Geometry check sheet. Reference: the model listing, model coordinates, mm. A direction names the side the tool comes from. Give positions to 0.01 mm unless a question says otherwise; leave off trailing zeros. Order: outer loops, then holes, each group sorted by start corner. A loop starts at its lowest first (then second) coordinate and runs counter-clockwise, first axis right, second up. Notation, with made-up numbers: M -34,-34.5 L -10,-34.5 A17 ccw -10,-5.5 Z; hole C -7.75,47 d2. An arc over 180 degrees is marked long. One line per question, with ' | ' between items. Start each with the question number.
Autodesk Inventor part; units mm, degrees
ref_plane "YZ Plane" through (0, 0, 0) normal (1, 0, 0) x (0, 1, 0)
ref_plane "XZ Plane" through (0, 0, 0) normal (0, 1, 0) x (-1, 0, 0)
ref_plane "XY Plane" through (0, 0, 0) normal (0, 0, 1) x (1, 0, 0)
sketch "Sketch1" plane through (0, 0, 0) normal (0, 0, 1) x (1, 0, 0)
  circle A0 centre (0, 0) radius 7.5
  arc A1 (6, -6.5) -> (6, 6.5) centre (6, 0) ccw
  line L0 (6, -6.5) -> (-6, -6.5)
  arc A2 (-6, 6.5) -> (-6, -6.5) centre (-6, 0) ccw
  line L1 (-6, 6.5) -> (6, 6.5)
  dimension "d0" = 15
  dimension "d6" = 6
  dimension "d8" = 6
  dimension "d22" = 6.5
  dimension "d23" = 6.5
  dimension "d24" = 12
extrude "Extrusion1" add sketch "Sketch1" along normal blind 3
sketch "草圖4" plane through (0, 0, 3) normal (0, 0, 1) x (1, 0, 0)
  arc A0 (3.7417, 6.5) -> (-3.7417, 6.5) centre (0, 0) ccw
  line L0 (1.3279, 2.3) -> (2.6558, 0)
  line L1 (2.6558, 0) -> (1.3279, -2.3)
  line L2 (1.3279, -2.3) -> (-1.3279, -2.3)
  line L3 (-1.3279, -2.3) -> (-2.6558, 0)
  line L4 (-2.6558, 0) -> (-1.3279, 2.3)
  line L5 (-1.3279, 2.3) -> (1.3279, 2.3)
  point P0 (-2.7439, 4.7667)
  point P1 (2.7439, 4.7667)
  point P2 (-6, -4.5)
  point P3 (6, -4.5)
  dimension "d17" = 4.6
extrude "擠出2" cut sketch "草圖4" against normal through all
fillet "圓角2" radius 4 4 edges at (3.7417, -6.5, 1.5) (-3.7417, -6.5, 1.5) (3.7417, 6.5, 1.5) (-3.7417, 6.5, 1.5)
sketch "草圖5" plane through (0, 0, 3) normal (0, 0, 1) x (1, 0, 0)
  arc A0 (6, -6.5) -> (6, 6.5) centre (6, 0) ccw
  arc A1 (-6, 6.5) -> (-6, -6.5) centre (-6, 0) ccw
hole "孔2" at (-6, 0, 3) at (6, 0, 3) direction (0, 0, -1) diameter 3 end through all
properties part number "plastic_part_99"
Item 1: Cross-section at D-D, the plane x = 10.5. Record the cut outline in (y, z), plus the area to 3 significant figures.
Item 2: Cross-section at A-A, the plane z = 1.55. Record the cut outline in (x, y), plus the area to 3 significant figures.
Item 3: Cross-section at C-C, the plane x = -1.75. Record the cut outline in (y, z).
Item 4: Material ranges on line 1 along Y through (x, z) = (-6, 2.1); line 2 along X through (y, z) = (0.5, 2.05); line 3 along Y through (x, z) = (1.5, 1.85), recorded low to high.
Item 5: Depth check by flat-ended pin: pin 1 (1.4 mm diameter, centred on x = 5, z = 1.5, fed in from +Y); pin 2 (1.4 mm diameter, centred on x = 5, z = 1, fed in from -Y). Enter the tip coordinate at first touch or a pass-through.
Item 6: Cross-section at B-B, the plane y = 1.25. Record the cut outline in (x, z), plus the area to 3 significant figures.
Item 7: Set-up check for faces 4 (the flat face through (5, 6.5, 1)), 5 (the flat face through (-2.001, 1.134, 1.521)), 6 (the flat face through (-5, -6.5, 1)): record each of +Z, -Z, +X, -X, +Y, -Y from which the full face is reachable in a straight line by a thin tool's end or side.
Item 8: Mould release check, pull along X, two halves, no side actions. Record for faces 1 (the cylindrical face through (3.8, 6.6, 1.5)), 2 (the flat face through (-3, 0, 0)), 3 (the cylindrical face through (7.464, 0.325, 1.479)): released by +X, released by -X, zero draft, split by the parting line, or undercut.
Outcome:
1) outline: M -4.69,0 L 4.69,0 L 4.69,3 L -4.69,3 Z | area: 28.1 mm²
2) outline: M -6,-6.5 L -4.69,-6.5 A4 cw -3.06,-6.85 A7.5 ccw 3.06,-6.85 A4 cw 4.69,-6.5 L 6,-6.5 A6.5 ccw 6,6.5 L 4.69,6.5 A4 cw 3.06,6.85 A7.5 ccw -3.06,6.85 A4 cw -4.69,6.5 L -6,6.5 A6.5 ccw Z; hole C -6,0 d3; hole M -2.66,0 L -1.33,-2.3 L 1.33,-2.3 L 2.66,0 L 1.33,2.3 L -1.33,2.3 Z; hole C 6,0 d3 | area: 267 mm²
3) outline: M -7.29,0 L -1.57,0 L -1.57,3 L -7.29,3 Z; M 1.57,0 L 7.29,0 L 7.29,3 L 1.57,3 Z
4) line 1: y = -6.5 to -1.5, 1.5 to 6.5 | line 2: x = -12.48 to -7.41, -4.59 to -2.37, 2.37 to 4.59, 7.41 to 12.48 | line 3: y = -7.35 to -2, 2 to 7.35
5) pin 1: stops at y = 6.52 | pin 2: stops at y = -6.52
6) outline: M -12.38,0 L -6.83,0 L -6.83,3 L -12.38,3 Z; M -5.17,0 L -1.93,0 L -1.93,3 L -5.17,3 Z; M 1.93,0 L 5.17,0 L 5.17,3 L 1.93,3 Z; M 6.83,0 L 12.38,0 L 12.38,3 L 6.83,3 Z | area: 52.7 mm²
7) face 4: +Z, -Z, +X, +Y | face 5: +Z, -Z | face 6: +Z, -Z, -X, -Y
8) face 1: released by +X | face 2: zero draft | face 3: undercut
